Study the drawing (mm; zero at the part's minimum x, y, z) and answer. Coordinates: 2 decimals unless noted, no trailing zeros. Write each loop counter-clockwise with the first axis right and the second up, starting at its lowest first coordinate (ties: lowest second). Pieces come first, ordered by that corner, then holes. Notation, with made-up numbers: (-4.75, -28.75) -> (46.25, -28.75) arc R27 cw to (46.25, -0.75) -> close; hole circle Ø7 at (9.25, -16.5). An arc over 180 degrees is marked (long way). Answer in a Markdown table with one row per item. Add a question column.
Item 1: Section B-B on z = 65.5 is taken. Write down the section's boundary in (x, y), then the cut area to 3 significant figures.
Item 2: Section D-D on x = 22 is taken. Write down the section's boundary in (y, z).
Item 3: Straight lines are drawn through the part: line 1 (X direction, y = 3.05, z = 28); line 2 (Z direction, x = 30, y = 2); line 3 (Z direction, x = 27, y = 1.85). For each, find the intervals that lie inside material, in ascending order. Write a range as from..to.
Item 4: Section C-C on y = 0.75 is taken. Write down the section's boundary in (x, z).
Item 5: Given pin 1 Ø10.5 at (x, z) = (30, 85.5) entering from -Y; pin 2 Ø4.5 at (x, z) = (30, 10) entering from -Y, each flat-ended and moving along its own axis, determine where each tip first touches the part or whether it passes through.
Item 6: Section A-A on x = 30 is taken. Write down the section's boundary in (y, z), then the cut area to 3 significant figures.
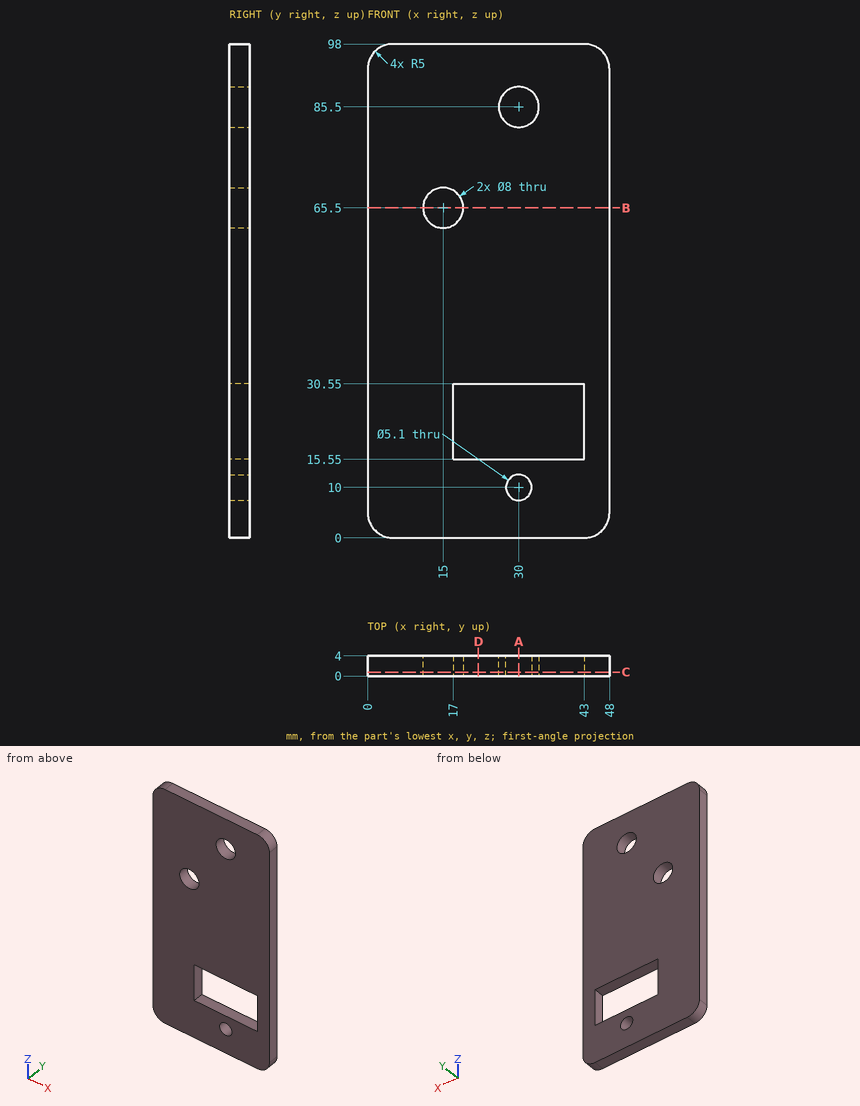
Results below:
| question | item | result |
|---|---|---|
| 1 | outline | (0, 0) -> (11, 0) -> (11, 4) -> (0, 4) -> close; (19, 0) -> (48, 0) -> (48, 4) -> (19, 4) -> close |
| 1 | area | 160 mm2 |
| 2 | outline | (0, 0) -> (4, 0) -> (4, 15.55) -> (0, 15.55) -> close; (0, 30.55) -> (4, 30.55) -> (4, 98) -> (0, 98) -> close |
| 3 | line 1 | x = 0..17, 43..48 |
| 3 | line 2 | z = 0..7.45, 12.55..15.55, 30.55..81.5, 89.5..98 |
| 3 | line 3 | z = 0..15.55, 30.55..82.85, 88.15..98 |
| 4 | outline | (0, 5) arc R5 ccw to (5, 0) -> (43, 0) arc R5 ccw to (48, 5) -> (48, 93) arc R5 ccw to (43, 98) -> (5, 98) arc R5 ccw to (0, 93) -> close; hole circle Ø8 at (15, 65.5); hole (17, 15.55) -> (43, 15.55) -> (43, 30.55) -> (17, 30.55) -> close; hole circle Ø8 at (30, 85.5); hole circle Ø5.1 at (30, 10) |
| 5 | pin 1 | stops at y = 0 |
| 5 | pin 2 | passes through |
| 6 | outline | (0, 0) -> (4, 0) -> (4, 7.45) -> (0, 7.45) -> close; (0, 12.55) -> (4, 12.55) -> (4, 15.55) -> (0, 15.55) -> close; (0, 30.55) -> (4, 30.55) -> (4, 81.5) -> (0, 81.5) -> close; (0, 89.5) -> (4, 89.5) -> (4, 98) -> (0, 98) -> close |
| 6 | area | 280 mm2 |
